Here's how the part is built. I have some questions about the finished solid (model axes, mm). A direction names the side the tool comes from. Coordinates: 2 decimals unless noted, no trailing zeros. Write each loop counter-clockwise with the first axis right and the second up, starting at its lowest first coordinate (ties: lowest second). Pieces come first, ordered by that corner, then holes.
(1) Please list where these lines run through material, in increasing order: probe 1 along Z at (x, y) = (3.5, 1); probe 2 along Z at (x, y) = (-1, -2.5); probe 3 along Y at (x, z) = (1.5, 20).
(2) For pin 1 Ø3 at (x, z) = (3, -5.5) entering from -Y; pin 2 Ø1 at (x, z) = (0, 64.5) entering from +Y; pin 3 Ø0.5 at (y, z) = (3, 64.5) entering from -X, each with a flat end and sliding along its axis, tell me the tip position at first contact or that it passes through.
(3) Which directions (+Z, -Z, +X, -X, +Y, -Y) give clear straight access to the entire face, cutting with the end or side of a thin tool? Please do faces 1 (the cylindrical face through (-0.705, -3.173, 58.971)), 2 (the flat face through (1.1, -1.1, -66)), 3 (the cylindrical face through (3, 0, -60)).
(4) Imagine slicing it at A-A, the plane z = -37.5. List the corners of the cut face in (x, y) for me, plus the area to 3 significant figures.
(5) Thinking about a two-plate mould opening in Y: for faces 4 (the flat face through (0, 2.5, 64)), 5 (the flat face through (0, 0, -61)), 6 (the flat face through (-2, 3, 52)), 7 (the cylindrical face through (0.54, -2.44, -63.54)), which applies, released by +Y, released by -Y, zero draft, split by the parting line, or undercut?
```python
from build123d import *

# Parameters (mm, degrees)
SKETCH1_R           = 4
BOSS_EXTRUDE1_DEPTH = 66
SKETCH2_R           = 4
SKETCH2_R_2         = 3.25
CUT_EXTRUDE1_DEPTH  = 14
CUT_EXTRUDE2_DEPTH  = 1
CHAMFER1_SIZE       = 0.25
CUT_EXTRUDE3_START  = -7
SKETCH5_R           = 4
SKETCH5_R_2         = 3
CUT_EXTRUDE3_DEPTH  = 7
SKETCH7_R           = 3.566008396
SKETCH7_R_2         = 2.5
CUT_EXTRUDE4_DEPTH  = 5
CUT_EXTRUDE5_DEPTH  = 5


with BuildPart() as part:
    # Sketch1 → Boss-Extrude1 (new, symmetric)
    with BuildSketch(Plane.XY):
        Circle(SKETCH1_R)
    extrude(amount=BOSS_EXTRUDE1_DEPTH, both=True)

    # Sketch2 → Cut-Extrude1 (cut)
    with BuildSketch(Plane.XY.offset(66)):
        Circle(SKETCH2_R)
        Circle(SKETCH2_R_2, mode=Mode.SUBTRACT)
    extrude(amount=-CUT_EXTRUDE1_DEPTH, mode=Mode.SUBTRACT)

    # Sketch3 → Cut-Extrude2 (cut)
    with BuildSketch(Plane(origin=(0, 3.5, 0), x_dir=(1, 0, 0), z_dir=(0, 1, 0))):
        with BuildLine():
            Line((1, -62.5), (1, -66))
            ThreePointArc((1, -66), (0, -67), (-1, -66))
            Line((-1, -66), (-1, -62.5))
            ThreePointArc((-1, -62.5), (0, -61.5), (1, -62.5))
        make_face()
    extrude(amount=-CUT_EXTRUDE2_DEPTH, mode=Mode.SUBTRACT)

    # Chamfer1
    chamfer1_edges = [part.edges().sort_by_distance(p)[0] for p in [
        (-1.912132318, -2.627974505, 66),
    ]]
    chamfer(chamfer1_edges, length=CHAMFER1_SIZE)

    # Sketch5 → Cut-Extrude3 (cut)
    with BuildSketch(Plane(origin=(0, 0, -66), x_dir=(-1, 0, 0), z_dir=(0, 0, -1)).offset(CUT_EXTRUDE3_START)):
        Circle(SKETCH5_R)
        Circle(SKETCH5_R_2, mode=Mode.SUBTRACT)
    extrude(amount=CUT_EXTRUDE3_DEPTH, mode=Mode.SUBTRACT)

    # Sketch7 → Cut-Extrude4 (cut)
    with BuildSketch(Plane(origin=(0, 0, -66), x_dir=(-1, 0, 0), z_dir=(0, 0, -1))):
        Circle(SKETCH7_R)
        Circle(SKETCH7_R_2, mode=Mode.SUBTRACT)
    extrude(amount=-CUT_EXTRUDE4_DEPTH, mode=Mode.SUBTRACT)

    # Sketch8 → Cut-Extrude5 (cut)
    with BuildSketch(Plane(origin=(0, 0, -66), x_dir=(-1, 0, 0), z_dir=(0, 0, -1))):
        Polygon((0.75, -1.299038106), (1.5, 0), (0.75, 1.299038106), (-0.75, 1.299038106), (-1.5, 0), (-0.75, -1.299038106), align=None)
    extrude(amount=-CUT_EXTRUDE5_DEPTH, mode=Mode.SUBTRACT)


solid = part.part
```
Recorded:
1. probe 1: z = -59 to 52
1. probe 2: z = -61 to 66
1. probe 3: y = -3.71 to 3.71
2. pin 1: stops at y = -3.71
2. pin 2: stops at y = 2.5
2. pin 3: stops at x = -1.73
3. face 1: +Z
3. face 2: -Z, +X, -X, +Y, -Y
3. face 3: -Z
4. outline: circle Ø8 at (0, 0)
4. area: 50.3 mm2
5. face 4: released by +Y
5. face 5: undercut
5. face 6: zero draft
5. face 7: split by the parting line
